from build123d import *

# Parameters (mm, degrees)
SKETCH_1_W          = 23
SKETCH_1_H          = 27.5
SKETCH_1_R          = 2.6
SKETCH_1_R_2        = 2
EXTRUDE_1_DEPTH     = 20
SKETCH_3_R          = 4.75
CUT_EXTRUDE_3_DEPTH = 16
SKETCH_2_R          = 1.6
EXTRUDE_2_DEPTH     = 5
FILLET_1_R          = 10


with BuildPart() as part:
    # 草图1 → 凸台-拉伸1 (new body)
    with BuildSketch(Plane.XY):
        with Locations((-3.5, 0)):
            Rectangle(SKETCH_1_W, SKETCH_1_H)
        with Locations((0, 9.25)):
            Circle(SKETCH_1_R, mode=Mode.SUBTRACT)
        with Locations(Location((0, -9.25, 0), (0, 0, 180))):
            Circle(SKETCH_1_R, mode=Mode.SUBTRACT)
        Circle(SKETCH_1_R_2, mode=Mode.SUBTRACT)
    extrude(amount=EXTRUDE_1_DEPTH)

    # 草图3 → 切除-拉伸3 (cut)
    with BuildSketch(Plane.XY.offset(20)):
        with Locations((0, 9.25)):
            Circle(SKETCH_3_R)
        with Locations((0, -9.25)):
            Circle(SKETCH_3_R)
    extrude(amount=-CUT_EXTRUDE_3_DEPTH, mode=Mode.SUBTRACT)

    # 草图2 → 凸台-拉伸2 (add)
    with BuildSketch(Plane.ZY.offset(15)):
        with BuildLine():
            Line((0, 13.75), (20, 13.75))
            Line((20, 13.75), (29.338481678, 27.771599764))
            ThreePointArc((29.338481678, 27.771599764), (33.767848759, 29.99282055), (37.93415499, 27.310469546))
            Line((37.93415499, 27.310469546), (45, 13.75))
            Line((45, 13.75), (45, -13.75))
            Line((45, -13.75), (37.93415499, -27.310469546))
            ThreePointArc((37.93415499, -27.310469546), (33.767848759, -29.99282055), (29.338481678, -27.771599764))
            Line((29.338481678, -27.771599764), (20, -13.75))
            Line((20, -13.75), (0, -13.75))
            Line((0, -13.75), (0, 13.75))
        make_face()
        with Locations((33.5, 25)):
            Circle(SKETCH_2_R, mode=Mode.SUBTRACT)
        with Locations((33.5, -25)):
            Circle(SKETCH_2_R, mode=Mode.SUBTRACT)
    extrude(amount=EXTRUDE_2_DEPTH)

    # 圆角1
    fillet_1_edges = [part.edges().sort_by_distance(p)[0] for p in [
        (-17.5, -13.75, 20),
        (-17.5, -13.75, 45),
        (-17.5, 13.75, 45),
        (-17.5, 13.75, 20),
    ]]
    fillet(fillet_1_edges, radius=FILLET_1_R)


solid = part.part
Verification items for the finished model (mm, model axes). A direction names the side the tool comes from. Give positions to 0.01 mm unless a question says otherwise; leave off trailing zeros. Write each loop counter-clockwise with the first axis right and the second up, starting at its lowest first coordinate (ties: lowest second). Pieces come first, ordered by that corner, then holes. Notation, with made-up numbers: (59, 49) -> (90, 49) arc R25 ccw to (90, 80) -> close; hole circle Ø5 at (7.5, 79). An arc over 180 degrees is marked (long way). Use CSV: the item, a comma, the result in double quotes.
(1) Sectioned sample at A-A (y = 0). Record the cut outline in (x, z), plus the area to 3 significant figures.
Derived:
outline,"(-20, 0) -> (-2, 0) -> (-2, 20) -> (-15, 20) -> (-15, 45) -> (-20, 45) -> close; (2, 0) -> (8, 0) -> (8, 20) -> (2, 20) -> close"
area,"605 mm^2"
(2) Sectioned sample at B-B (z = 33.5). Record the cut outline in (x, y).
Derived:
outline,"(-20, -30) -> (-15, -30) -> (-15, -26.6) -> (-20, -26.6) -> close; (-20, -23.4) -> (-15, -23.4) -> (-15, 23.4) -> (-20, 23.4) -> close; (-20, 26.6) -> (-15, 26.6) -> (-15, 30) -> (-20, 30) -> close"
(3) Sectioned sample at D-D (y = 25). Record the cut outline in (x, z).
Derived:
outline,"(-20, 27.49) -> (-15, 27.49) -> (-15, 31.9) -> (-20, 31.9) -> close; (-20, 35.1) -> (-15, 35.1) -> (-15, 39.14) -> (-20, 39.14) -> close"
(4) Set-up check for faces 1 (the flat face through (2.04, -11.12, 4)), 2 (the flat face through (-6, -13.75, 10)), 3 (the flat face through (-4, 0, 20)), 4 (the flat face through (-6, 13.75, 10)): record each of +Z, -Z, +X, -X, +Y, -Y from which the full face is reachable in a straight line by a thin tool's end or side.
Derived:
face 1,"+Z"
face 2,"-Z, +X, -Y"
face 3,"+Z, +X, +Y, -Y"
face 4,"-Z, +X, +Y"
(5) Material ranges on L1, parallel to Y at x = 0, z = 2.6; L2, parallel to Y at x = -18.4, z = 33.5; L3, parallel to X at y = 9.25, z = 15.75, recorded low to high.
Derived:
L1,"y = -13.75 to -11.85, -6.65 to -2, 2 to 6.65, 11.85 to 13.75"
L2,"y = -30 to -26.6, -23.4 to 23.4, 26.6 to 30"
L3,"x = -20 to -4.75, 4.75 to 8"
(6) Go/stop test with flat-tipped pins: pin 1 (24.5 mm diameter, centred on y = 13, z = 35.5, fed in from +X); pin 2 (3 mm diameter, centred on x = 2, y = -11, fed in from +Z); pin 3 (12 mm diameter, centred on x = 1.5, z = 23, fed in from -Y). Record where each tip stops, or that it passes through.
Derived:
pin 1,"stops at x = -15"
pin 2,"stops at z = 4"
pin 3,"stops at y = -13.75"
(7) Release check for a two-part mould opening along Z. For faces 5 (the cylindrical face through (-17.46, -23.92, 32.32)), 6 (the cylindrical face through (-17.46, 25.07, 31.9)), 7 (the cylindrical face through (0.187, -4.504, 12.112)), 8 (the cylindrical face through (-17.5, -14.9, 19.3)) record: +Z half, -Z half, draft (parallel to the pull), parting line (faces both ways), or undercut.
Derived:
face 5,"undercut"
face 6,"undercut"
face 7,"draft"
face 8,"-Z half"
(8) Sectioned sample at C-C (x = -9.5). Record the cut outline in (y, z).
Derived:
outline,"(-13.75, 0) -> (13.75, 0) -> (13.75, 20) -> (-13.75, 20) -> close"
